Autodesk Inventor part; units mm, degrees
ref_plane "YZ Plane" through (0, 0, 0) normal (1, 0, 0) x (0, 1, 0)
ref_plane "XZ Plane" through (0, 0, 0) normal (0, 1, 0) x (-1, 0, 0)
ref_plane "XY Plane" through (0, 0, 0) normal (0, 0, 1) x (1, 0, 0)
sketch "スケッチ1" plane through (0, 0, 0) normal (0, 0, 1) x (1, 0, 0)
  line L0 (-15.75, -60) -> (15.75, -60)
  line L1 (15.75, -60) -> (15.75, 60)
  line L2 (15.75, 60) -> (-15.75, 60)
  line L3 (-15.75, 60) -> (-15.75, -60)
  point P0 (0, 0)
  dimension "d0" = 31.5
  dimension "d1" = 15.75
  dimension "d2" = 120
  dimension "d3" = 60
extrude "押し出し1" add sketch "スケッチ1" along normal blind 5
fillet "フィレット1" radius 15.75 4 edges at (-15.75, 60, 2.5) (15.75, 60, 2.5) (15.75, -60, 2.5) (-15.75, -60, 2.5)
sketch "スケッチ2" plane through (0, 0, 5) normal (0, 0, 1) x (1, 0, 0)
  arc A0 (15.75, 44.25) -> (-15.75, 44.25) centre (0, 44.25) ccw
  circle A1 centre (0, 44.25) radius 11.25
  point P0 (0, 0)
  point P1 (0, 55.5)
  point P2 (9.7428, 49.875)
  point P3 (9.7428, 38.625)
  point P4 (0, 33)
  point P5 (-9.7428, 38.625)
  point P6 (-9.7428, 49.875)
  dimension "d7" = 22.5
  dimension "d10" = 360
hole "Hole1" at (0, 55.5, 5) at (9.7428, 49.875, 5) at (9.7428, 38.625, 5) at (0, 33, 5) at (-9.7428, 38.625, 5) at (-9.7428, 49.875, 5) direction (0, 0, -1) diameter 1.567 depth 8 tip angle 118
sketch "スケッチ3" plane through (0, 0, 5) normal (0, 0, 1) x (1, 0, 0)
  arc A0 (15.75, 44.25) -> (-15.75, 44.25) centre (0, 44.25) ccw
  point P0 (0, 0)
hole "Hole2" at (0, 44.25, 5) direction (0, 0, -1) diameter 13 end through all
chamfer "面取り1" distance 1 distance2 5 1 edges at (0, 50.75, 5) measured on face at (0, -18.7612, 5)
sketch "スケッチ5" plane through (0, 0, 0) normal (0, 0, -1) x (-1, 0, 0)
  circle A0 centre (9.7428, 49.875) radius 0.7835
  circle A1 centre (9.7428, 38.625) radius 0.7835
  circle A2 centre (0, 33) radius 0.7835
  circle A3 centre (-9.7428, 38.625) radius 0.7835
  circle A4 centre (-9.7428, 49.875) radius 0.7835
  circle A5 centre (0, 55.5) radius 0.7835
  arc A6 (-15.75, -44.25) -> (15.75, -44.25) centre (0, -44.25) ccw
  line L0 (15.75, 44.25) -> (15.75, -44.25)
  arc A7 (15.75, 44.25) -> (-15.75, 44.25) centre (0, 44.25) ccw
  line L1 (-15.75, -44.25) -> (-15.75, 44.25)
  circle A8 centre (0, 44.25) radius 3
  point P0 (0, 0)
  dimension "d31" = 6
extrude "押し出し3" add sketch "スケッチ5" along normal blind 15
sketch "スケッチ6" plane through (0, 44.25, 0) normal (0, 0, 1) x (1, 0, 0)
  circle A0 centre (0, 0) radius 3
  circle A1 centre (0, 0) radius 6.5
  point P0 (0, -44.25)
extrude "押し出し4" cut sketch "スケッチ6" against normal blind 1
sketch "スケッチ7" plane through (0, 44.25, -1) normal (0, 0, 1) x (1, 0, 0)
  circle A0 centre (0, 0) radius 6.5
  circle A1 centre (0, 0) radius 4.5
  point P0 (0, -44.25)
  dimension "d36" = 9
extrude "押し出し5" cut sketch "スケッチ7" against normal blind 1
fillet "フィレット2" radius 1 2 edges at (-6.5, 44.25, -2) (-4.5, 44.25, -2)
sketch "スケッチ9" plane through (0, 0, 5) normal (0, 0, 1) x (1, 0, 0)
  arc A0 (-15.75, -44.25) -> (15.75, -44.25) centre (0, -44.25) ccw
  line L0 (15.75, 44.25) -> (15.75, -44.25)
  arc A1 (15.75, 44.25) -> (-15.75, 44.25) centre (0, 44.25) ccw
  line L1 (-15.75, -44.25) -> (-15.75, 44.25)
  circle A2 centre (0, 44.25) radius 7.5
  circle A3 centre (0, 44.25) radius 13.9
  point P0 (0, 0)
  dimension "d46" = 27.8
extrude "押し出し7" cut sketch "スケッチ9" against normal blind 6 contours L1 A1 L0 A0
sketch "スケッチ10" plane through (0, 0, -1) normal (0, 0, 1) x (1, 0, 0)
  line L0 (15.75, 44.25) -> (15.75, -44.25)
  arc A0 (15.75, 44.25) -> (-15.75, 44.25) centre (0, 44.25) ccw
  line L1 (-15.75, -44.25) -> (-15.75, 44.25)
  arc A1 (-15.75, -44.25) -> (15.75, -44.25) centre (0, -44.25) ccw
  arc A2 (15.75, 24.8351) -> (-15.75, 24.8351) centre (0, 44.25) ccw
  arc A3 (-15.75, 24.8351) -> (15.75, 24.8351) centre (0, 44.25) ccw
  point P0 (0, 0)
  dimension "d49" = 50
extrude "押し出し8" cut sketch "スケッチ10" against normal blind 10 contours L0 A1 L1 A3
sketch "スケッチ11" plane through (0, 0, -11) normal (0, 0, 1) x (1, 0, 0)
  arc A0 (-15.75, -44.25) -> (15.75, -44.25) centre (0, -44.25) ccw
  point P0 (0, 0)
hole "Hole3" at (0, -44.25, -11) direction (0, 0, -1) diameter 4 end through all
sketch "スケッチ12" plane through (0, 0, -1) normal (0, 0, 1) x (1, 0, 0)
  line L0 (-15.75, 24.8351) -> (-15.75, 44.25)
  circle A0 centre (0, 44.25) radius 13.9
  circle A1 centre (0, 44.25) radius 19.5
  line L1 (0, 44.25) -> (0, 63.75)
  line L2 (0, 44.25) -> (-9.75, 27.3625)
  line L3 (0, 44.25) -> (9.75, 27.3625)
  line L4 (15.75, 44.25) -> (15.75, 24.8351)
  arc A2 (15.75, 44.25) -> (-15.75, 44.25) centre (0, 44.25) ccw
  line L5 (0, 44.25) -> (0, 24.75)
  point P0 (0, 0)
  dimension "d59" = 39
  dimension "d60" = 150
  dimension "d61" = 150
hole "Hole4" at (-9.75, 27.3625, -1) at (9.75, 27.3625, -1) at (0, 24.75, -1) direction (0, 0, -1) diameter 2.459 end through all
sketch "スケッチ14" plane through (0, 0, -11) normal (0, 0, 1) x (1, 0, 0)
  circle A0 centre (0, -44.25) radius 2
  arc A1 (-15.75, 24.8351) -> (15.75, 24.8351) centre (0, 44.25) ccw
  arc A2 (-15.75, -44.25) -> (15.75, -44.25) centre (0, -44.25) ccw
  line L0 (-9.85, 12.8) -> (9.85, 12.8)
  line L1 (9.85, 12.8) -> (9.85, -23.1)
  line L2 (9.85, -23.1) -> (-9.85, -23.1)
  line L3 (-9.85, -23.1) -> (-9.85, 12.8)
  line L4 (0, 19.25) -> (0, -60)
  point P0 (0, 0)
  dimension "d77" = 19.7
  dimension "d78" = 19.7
  dimension "d79" = 35.9
  dimension "d80" = 21.15
extrude "押し出し9" cut sketch "スケッチ14" against normal through all contours L0 L4 L2 L3 | L0 L1 L2 L4
fillet "フィレット3" radius 5.05 2 edges at (-9.85, -23.1, -13) (9.85, -23.1, -13)
fillet "フィレット4" radius 3.05 2 edges at (-9.85, 12.8, -13) (9.85, 12.8, -13)
sketch "スケッチ15" plane through (0, 0, -11) normal (0, 0, 1) x (1, 0, 0)
  line L0 (-6.8, 12.8) -> (6.8, 12.8)
  circle A0 centre (0, -44.25) radius 2
  line L1 (15.75, 24.8351) -> (15.75, -44.25)
  circle A1 centre (0, 44.25) radius 31.45
  line L2 (0, 19.25) -> (0, 12.8)
  circle A2 centre (0, 44.25) radius 28.225
  line L3 (0, 44.25) -> (0, 12.8)
  line L4 (0, 44.25) -> (-11.9284, 18.6695)
  line L5 (0, 44.25) -> (11.9284, 18.6695)
  circle A3 centre (0, -44.25) radius 12.5
  line L6 (0, -44.25) -> (0, -56.75)
  line L7 (0, -44.25) -> (10.8253, -50.5)
  line L8 (0, -44.25) -> (-10.8253, -50.5)
  point P0 (0, 0)
  point P1 (0, 16.025)
  point P2 (10.8253, -50.5)
  dimension "d86" = 25
  dimension "d87" = 25
  dimension "d88" = 25
  dimension "d93" = 120
  dimension "d94" = 60
  dimension "d95" = 180
  dimension "d96" = 0
  dimension "d97" = 0
hole "Hole6" at (0, -44.25, -11) at (-11.9284, 18.6695, -11) at (0, 16.025, -11) at (11.9284, 18.6695, -11) at (10.8253, -50.5, -11) at (0, -56.75, -11) at (-10.8253, -50.5, -11) direction (0, 0, -1) diameter 1.567 depth 8 tip angle 118
chamfer "面取り2" distance 0.5 angle 45 4 edges at (-15.75, 0, -15) (0, -60, -15) (15.75, 0, -15) (0, 60, -15)
equation "\"d60\" = d61"
equation "\"d78\" = d77"
equation "\"d94\" = 0.5 * d93"
properties part number "JointC2_2nd" material "ポリプロピレン"
For this review, take the finished solid that the model builds, in its own axes (mm). A direction names the side the tool comes from. Give positions to 0.01 mm unless a question says otherwise; leave off trailing zeros. Loops run counter-clockwise (first coordinate to the right, second up) from the corner with the lowest first, then second, coordinate; pieces in that order, holes last.
Item 1: Take a section at C-C, the plane y = -31. State the section outline as (x, z) points, and give its area (3 significant figures).
Item 2: Take a section at B-B, the plane z = -9. Give the number of separate pieces and of enclosed holes in the cut face, and give its area (3 significant figures).
Item 3: Draft analysis for pull direction Y (two halves, no side actions). For faces 5 (the flat face through (-10, 1, -15)), 6 (the cylindrical face through (0.391, 41.276, -7.902)), 7 (the conical face through (0.338, 59.639, -14.858)), state which applies: +Y half, -Y half, draft (parallel to the pull), parting line (faces both ways), or undercut.
Item 4: Take a section at A-A, the plane y = 1. State the section outline as (x, z) points.
Item 5: For line 1 along Y through (x, z) = (0, -0.25); line 2 along X through (y, z) = (-50.5, -13.8); line 3 along Y through (x, z) = (9.5, -3.25), list the stretches that pass through material, from the lowest coordinate up.
Item 6: Tool access review of faces 1 (the cylindrical face through (-0.24, 19.25, -5.93)), 2 (the flat face through (6, 38, 5)), 3 (the cylindrical face through (8.933, 11.93, -13.028)), 4 (the cylindrical face through (-1.409, 37.905, -0.493)): name each direction out of +Z, -Z, +X, -X, +Y, -Y from which nothing blocks a thin tool from reaching the whole face with its end or side.
Item 7: Insertion check: pin 1 (16 mm diameter, centred on x = -5.5, y = -35.5, fed in from +Z); pin 2 (4 mm diameter, centred on x = 6.5, z = -2, fed in from +Y); pin 3 (3 mm diameter, centred on y = 19, z = 1.5, fed in from +X); pin 4 (10.5 mm diameter, centred on x = 0, y = 44.25, fed in from +Z). Each pin has a flat end and moves straight along its axis. Give the tip position at first contact, or say it passes through.
Calculated:
1. outline: (-15.75, -14.5) - (-15.25, -15) - (15.25, -15) - (15.75, -14.5) - (15.75, -11) - (-15.75, -11) - close
1. area: 126 mm2
2. separate pieces: 1
2. enclosed holes: 10
2. area: 1,070 mm2
3. face 5: draft
3. face 6: undercut
3. face 7: +Y half
4. outline: (-15.75, -14.5) - (-15.25, -15) - (-9.85, -15) - (-9.85, -11) - (-15.75, -11) - close; (9.85, -15) - (15.25, -15) - (15.75, -14.5) - (15.75, -11) - (9.85, -11) - close
5. line 1: y = 30.35 to 32.22, 33.78 to 37.75, 50.75 to 54.72, 56.28 to 58.15
5. line 2: x = -14.46 to -11.61, -10.04 to 10.04, 11.61 to 14.46
5. line 3: y = 21.13 to 26.16, 28.57 to 37.88, 39.37 to 49.13, 50.62 to 56.81
6. face 1: +Z, -Y
6. face 2: +Z, +X, -X, +Y, -Y
6. face 3: +Z, -Z
6. face 4: +Z
7. pin 1: stops at z = -11
7. pin 2: stops at y = 59.34
7. pin 3: passes through
7. pin 4: stops at z = -1
